For this review, use the dimensioned drawing (mm, ordinates from the lowest corner) and the shaded views. Round coordinates to 2 decimals unless told otherwise and drop trailing zeros. Write each loop counter-clockwise with the first axis right and the second up, starting at its lowest first coordinate (ties: lowest second). Pieces come first, ordered by that corner, then holes.
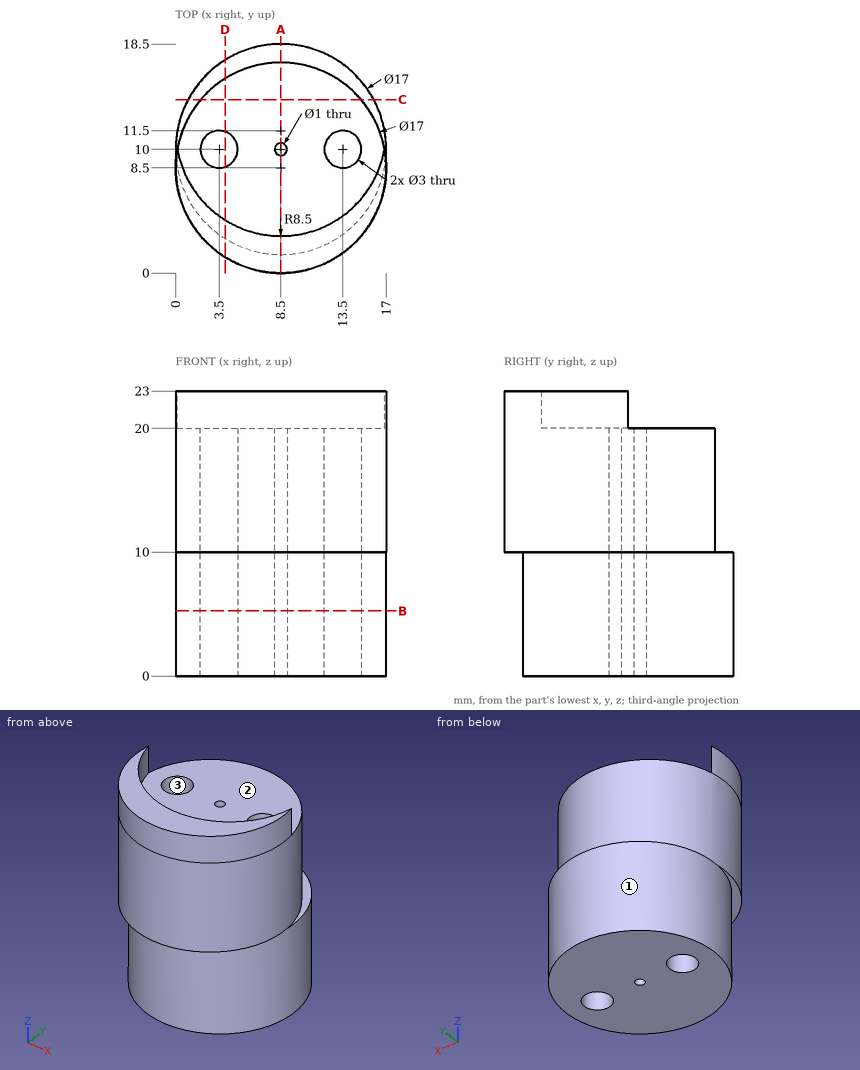
(1) We need section C-C, the plane y = 14. Give the boundary of the cut face in (x, z).
Geometry check:
outline: (1, 0) - (16, 0) - (16, 10) - (14.98, 10) - (14.98, 20) - (2.02, 20) - (2.02, 10) - (1, 10) - close
(2) For pin 1 Ø2 at (y, z) = (4, 9.5) entering from +X; pin 2 Ø4 at (x, y) = (13.5, 10) entering from +Z; pin 3 Ø8 at (x, z) = (14.5, 20.5) entering from -Y, all flat-tipped, find the tip position at first contact; note any pin that passes through.
Geometry check:
pin 1: stops at x = 16.18
pin 2: stops at z = 20
pin 3: stops at y = 0.24
(3) We need section B-B, the plane z = 5.25. Give the boundary of the cut face in (x, y), and give its area (3 significant figures).
Geometry check:
outline: circle Ø17 at (8.5, 10); hole circle Ø3 at (3.5, 10); hole circle Ø1 at (8.5, 10); hole circle Ø3 at (13.5, 10)
area: 212 mm2
(4) We need section A-A, the plane x = 8.5. Give the boundary of the cut face in (y, z).
Geometry check:
outline: (0, 10) - (1.5, 10) - (1.5, 0) - (9.5, 0) - (9.5, 20) - (3, 20) - (3, 23) - (0, 23) - close; (10.5, 0) - (18.5, 0) - (18.5, 10) - (17, 10) - (17, 20) - (10.5, 20) - close
(5) Mouldability with a two-part tool opening along Y and no side actions: class the marked faces 1, 2 and 3 as pulls with the +Y half, pulls with the -Y half, needs draft (parallel to the pull), parting line crosses it, or undercut.
Geometry check:
face 1: parting line crosses it
face 2: needs draft
face 3: undercut
(6) We need section D-D, the plane x = 4. Give the boundary of the cut face in (y, z).
Geometry check:
outline: (1.29, 10) - (2.79, 10) - (2.79, 0) - (8.59, 0) - (8.59, 20) - (4.29, 20) - (4.29, 23) - (1.29, 23) - close; (11.41, 0) - (17.21, 0) - (17.21, 10) - (15.71, 10) - (15.71, 20) - (11.41, 20) - close
(7) For line 1 along Y through (x, z) = (8.5, 16.25); line 2 along Z through (x, y) = (9.25, 17); line 3 along Z through (x, y) = (10.5, 11.75), list the stretches that pass through material, from the lowest coordinate up.
Geometry check:
line 1: y = 0 to 9.5, 10.5 to 17
line 2: z = 0 to 10
line 3: z = 0 to 20
